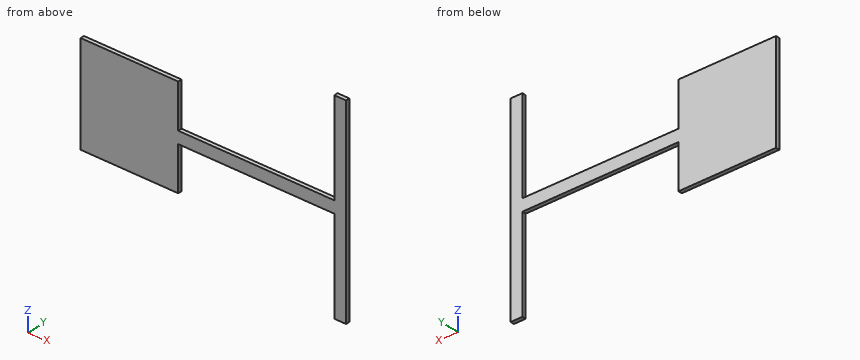
```python
from build123d import *

# Parameters (mm, degrees)
SKETCH1_W           = 250
SKETCH1_H           = 250
SKETCH1_W_2         = 400
SKETCH1_H_2         = 30
BOSS_EXTRUDE1_DEPTH = 10


with BuildPart() as part:
    # Sketch1 → Boss-Extrude1 (new body)
    with BuildSketch(Plane(origin=(0, 0, 0), x_dir=(1, 0, 0), z_dir=(0, 1, 0))):
        with Locations((-197.674418605, 16.472868217)):
            Rectangle(SKETCH1_W, SKETCH1_H)
        with Locations((127.325581395, 16.472868217)):
            Rectangle(SKETCH1_W_2, SKETCH1_H_2)
        Polygon((327.325581395, 266.472868217), (327.325581395, 31.472868217), (327.325581395, 1.472868217), (327.325581395, -233.527131783), (357.325581395, -233.527131783), (357.325581395, 266.472868217), align=None)
    extrude(amount=BOSS_EXTRUDE1_DEPTH)


solid = part.part
```
Check sheet for the modelled part. Datum: model origin and axes. Units: mm. Coordinates: 2 decimals unless noted, no trailing zeros. Write each loop counter-clockwise with the first axis right and the second up, starting at its lowest first coordinate (ties: lowest second). Pieces come first, ordered by that corner, then holes. Notation, with made-up numbers: M 73,-27 L 85,-27 A25 ccw 85,-4 Z; hole C 48,67.25 d6. An arc over 180 degrees is marked long. Use one line per item in the form item = value.
Item 1: Material ranges on L1, parallel to X at y = 6.75, z = 41.5; L2, parallel to Z at x = 173.5, y = 9.25; L3, parallel to X at y = 6, z = 154.5, recorded low to high. Write a range as from..to.
Answer below:
L1 = -322.67..-72.67, 327.33..357.33
L2 = -31.47..-1.47
L3 = 327.33..357.33
Item 2: Sectioned sample at D-D, the plane z = 127. Record the cut outline in (x, y).
Answer below:
outline = M 327.33,0 L 357.33,0 L 357.33,10 L 327.33,10 Z
Item 3: Sectioned sample at A-A, the plane z = 32. Record the cut outline in (x, y), and give its area (3 significant figures).
Answer below:
outline = M -322.67,0 L -72.67,0 L -72.67,10 L -322.67,10 Z; M 327.33,0 L 357.33,0 L 357.33,10 L 327.33,10 Z
area = 2,800 mm^2
Item 4: Gauge pin test, flat ends, axial feed: pin 1 Ø5 at (x, y) = (-229, 6.5) entering from -Z; pin 2 Ø3 at (x, y) = (60.5, 4) entering from -Z; pin 3 Ø4 at (x, y) = (157, 1) entering from +Z. Record the tip position at first contact, or that the pin passes through.
Answer below:
pin_1 = -141.47
pin_2 = -31.47
pin_3 = -1.47
Item 5: Sectioned sample at C-C, the plane x = -24. Record the cut outline in (y, z).
Answer below:
outline = M 0,-31.47 L 10,-31.47 L 10,-1.47 L 0,-1.47 Z
Item 6: Sectioned sample at B-B, the plane y = 5. Record the cut outline in (x, z).
Answer below:
outline = M -322.67,-141.47 L -72.67,-141.47 L -72.67,-31.47 L 327.33,-31.47 L 327.33,-266.47 L 357.33,-266.47 L 357.33,233.53 L 327.33,233.53 L 327.33,-1.47 L -72.67,-1.47 L -72.67,108.53 L -322.67,108.53 Z
